```python
from build123d import *

# Parameters (mm, degrees)
SKETCH1_W           = 175
SKETCH1_H           = 100
BOSS_EXTRUDE1_DEPTH = 80
SKETCH2_W           = 95
SKETCH2_H           = 25
CUT_EXTRUDE1_DEPTH  = 101
SKETCH3_W           = 56
SKETCH3_H           = 25
CUT_EXTRUDE2_DEPTH  = 176
SKETCH4_W           = 40
SKETCH4_H           = 30
CUT_EXTRUDE3_DEPTH  = 22


with BuildPart() as part:
    # Sketch1 → Boss-Extrude1 (new body)
    with BuildSketch(Plane(origin=(0, 0, 0), x_dir=(1, 0, 0), z_dir=(0, 1, 0))):
        Rectangle(SKETCH1_W, SKETCH1_H)
    extrude(amount=BOSS_EXTRUDE1_DEPTH)

    # Sketch2 → Cut-Extrude1 (cut, through all)
    with BuildSketch(Plane.XY.offset(50)):
        with Locations((0, 67.5)):
            Rectangle(SKETCH2_W, SKETCH2_H)
    extrude(amount=-CUT_EXTRUDE1_DEPTH, mode=Mode.SUBTRACT)

    # Sketch3 → Cut-Extrude2 (cut, through all)
    with BuildSketch(Plane(origin=(87.5, 0, 0), x_dir=(0, 0, -1), z_dir=(1, 0, 0))):
        with Locations((0, 67.5)):
            Rectangle(SKETCH3_W, SKETCH3_H)
    extrude(amount=-CUT_EXTRUDE2_DEPTH, mode=Mode.SUBTRACT)

    # Sketch4 → Cut-Extrude3 (cut)
    with BuildSketch(Plane.XY.offset(50)):
        with Locations((-67.5, 15)):
            Rectangle(SKETCH4_W, SKETCH4_H)
        with Locations((67.5, 15)):
            Rectangle(SKETCH4_W, SKETCH4_H)
    cut_extrude3 = extrude(amount=-CUT_EXTRUDE3_DEPTH, mode=Mode.SUBTRACT)

    # Mirror1: Cut-Extrude3 across plane
    add(cut_extrude3.mirror(Plane.XY), mode=Mode.SUBTRACT)


solid = part.part
```
Geometry check sheet. Reference: the model listing, model coordinates, mm. A direction names the side the tool comes from. Give positions to 0.01 mm unless a question says otherwise; leave off trailing zeros. Order: outer loops, then holes, each group sorted by start corner. A loop starts at its lowest first (then second) coordinate and runs counter-clockwise, first axis right, second up. Notation, with made-up numbers: (27, 86.25) - (72, 86.25) arc R33 ccw to (72, 120.25) - close; hole circle Ø1 at (-7, 18). An arc over 180 degrees is marked (long way). Write item = value, one per line. Start each with the question number.
1) Access from +Z, -Z, +X, -X, +Y, -Y to the whole of each face (thin tool, end or side, straight path). Record for faces 4 (the flat face through (67, 30, -39)), 5 (the flat face through (47.5, 67, 39)), 6 (the flat face through (-67, 67, -28)), 7 (the flat face through (-68, 30, 39)).
2) Draft check along X on faces 1 (the flat face through (-67, 67, 28)), 2 (the flat face through (87.5, 39, 1)), 3 (the flat face through (-47.5, 67, 39)). Enter one of: released by +X, released by -X, zero draft, split by the parting line, or undercut.
3) Scan lines: L1, parallel to X at y = 63.5, z = 40.5; L2, parallel to Z at x = 54, y = 71.5; L3, parallel to Y at x = 58.5, z = 36.5. Record each from-to range of solid material in increasing order.
4) Gauge pin test, flat ends, axial feed: pin 1 Ø12 at (x, z) = (25.5, 29.5) entering from +Y; pin 2 Ø6.5 at (x, z) = (-75, 35.5) entering from -Y; pin 3 Ø15 at (x, y) = (67, 9) entering from +Z. Record the tip position at first contact, or that the pin passes through.
5) Section check B-B (x = -50.5). Enter the section's corners in (y, z), then the cut area to 3 significant figures.
6) Section check D-D (z = 2). Enter the section's corners in (x, y).
7) Section check A-A (y = 65). Enter the section's corners in (x, z), then the cut area to 3 significant figures.
8) Section check C-C (z = -37). Enter the section's corners in (x, y).
Geometry check:
q1.face_4 = -Z, +X, -Y
q1.face_5 = +Z, -Z, +Y
q1.face_6 = +X, -X, +Y
q1.face_7 = +Z, -X, -Y
q2.face_1 = zero draft
q2.face_2 = released by +X
q2.face_3 = undercut
q3.L1 = -87.5 to -47.5, 47.5 to 87.5
q3.L2 = -50 to -28, 28 to 50
q3.L3 = 30 to 80
q4.pin_1 = 55
q4.pin_2 = 30
q4.pin_3 = 28
q5.outline = (0, -28) - (30, -28) - (30, -50) - (80, -50) - (80, -28) - (55, -28) - (55, 28) - (80, 28) - (80, 50) - (30, 50) - (30, 28) - (0, 28) - close
q5.area = 5,280 mm2
q6.outline = (-87.5, 0) - (87.5, 0) - (87.5, 55) - (-87.5, 55) - close
q7.outline = (-87.5, -50) - (-47.5, -50) - (-47.5, -28) - (-87.5, -28) - close; (-87.5, 28) - (-47.5, 28) - (-47.5, 50) - (-87.5, 50) - close; (47.5, -50) - (87.5, -50) - (87.5, -28) - (47.5, -28) - close; (47.5, 28) - (87.5, 28) - (87.5, 50) - (47.5, 50) - close
q7.area = 3,520 mm2
q8.outline = (-87.5, 30) - (-47.5, 30) - (-47.5, 0) - (47.5, 0) - (47.5, 30) - (87.5, 30) - (87.5, 80) - (47.5, 80) - (47.5, 55) - (-47.5, 55) - (-47.5, 80) - (-87.5, 80) - close
